```python
from build123d import *

# Parameters (mm, degrees)
SKETCH1_W               = 38.1
SKETCH1_H               = 15.875
BOSS_EXTRUDE1_DEPTH     = 7.62
SKETCH3_R               = 1.7
CUT_EXTRUDE1_DEPTH      = 49.4665
CUT_EXTRUDE2_DEPTH      = 3.302
CUT_EXTRUDE2_DEPTH_BACK = 22.2885
SKETCH4_R               = 1.7272


with BuildPart() as part:
    # Sketch1 → Boss-Extrude1 (new body)
    with BuildSketch(Plane.YZ):
        Rectangle(SKETCH1_W, SKETCH1_H)
    extrude(amount=BOSS_EXTRUDE1_DEPTH)

    # Sketch3 → Cut-Extrude1 (cut)
    with BuildSketch(Plane.XZ.offset(19.05)):
        with Locations(Location((4.36625, 0, 0), (0, 0, 270))):
            Circle(SKETCH3_R)
    extrude(amount=-CUT_EXTRUDE1_DEPTH, mode=Mode.SUBTRACT)

    # Sketch4 → Cut-Extrude2 (cut, two sides: drawn at the far end of the back side and taken through both)
    with BuildSketch(Plane.YZ.offset(7.62).offset(-CUT_EXTRUDE2_DEPTH_BACK)):
        with Locations(Location((-12.7, 4.7625, 0), (0, 0, 270))):
            Circle(SKETCH4_R)
        with Locations(Location((12.7, -4.7625, 0), (0, 0, 270))):
            Circle(SKETCH4_R)
    extrude(amount=CUT_EXTRUDE2_DEPTH + CUT_EXTRUDE2_DEPTH_BACK, mode=Mode.SUBTRACT)


solid = part.part
```
Part model, mm, in its own coordinate system. Round coordinates to 2 decimals unless told otherwise and drop trailing zeros. Write each loop counter-clockwise with the first axis right and the second up, starting at its lowest first coordinate (ties: lowest second). Pieces come first, ordered by that corner, then holes. Notation, with made-up numbers: (35.5, -9.75) -> (49.5, -9.75) arc R19 cw to (49.5, -0.75) -> close; hole circle Ø8 at (26.5, -9). An arc over 180 degrees is marked (long way). Return JSON: item names as keys, results as strings. Group by question number.
Q1. Saw through at C-C on z = 0. Write the cut outline in (x, y), plus the area to 3 significant figures.
Q2. Saw through at A-A on x = 5. Write the cut outline in (y, z), plus the area to 3 significant figures.
Q3. Mould opens along X. For faces 1 (the flat face through (7.62, 0, 0)), 2 (the flat face through (4, 0, 7.938)), 3 (the flat face through (0, 0, 0)), 4 (the cylindrical face through (5.52, -0.27, 1.25)) say: pulls with the +X half, pulls with the -X half, needs draft (parallel to the pull), parting line crosses it, or undercut.
Q4. Saw through at B-B on y = -11.5. Write the cut outline in (x, z), plus the area to 3 significant figures.
Q5. Saw through at D-D on x = 3.5. Write the cut outline in (y, z).
Q6. Probe L1, parallel to X at y = 7.5, z = 0; L2, parallel to Z at x = 5, y = 12.7; L3, parallel to Z at x = 4.5, y = -7. List the from-to ranges inside material, lowest first. Write a range as [from, to].
Answer:
{
 "1": {"outline": "(0, -19.05) -> (2.67, -19.05) -> (2.67, 19.05) -> (0, 19.05) -> close; (6.07, -19.05) -> (7.62, -19.05) -> (7.62, 19.05) -> (6.07, 19.05) -> close", "area": "161 mm2"},
 "2": {"outline": "(-19.05, -7.94) -> (19.05, -7.94) -> (19.05, -1.58) -> (-19.05, -1.58) -> close; (-19.05, 1.58) -> (19.05, 1.58) -> (19.05, 7.94) -> (-19.05, 7.94) -> close; hole circle Ø3.45 at (-12.7, 4.76); hole circle Ø3.45 at (12.7, -4.76)", "area": "466 mm2"},
 "3": {"face 1": "pulls with the +X half", "face 2": "needs draft", "face 3": "pulls with the -X half", "face 4": "undercut"},
 "4": {"outline": "(0, -7.94) -> (7.62, -7.94) -> (7.62, 3.52) -> (0, 3.52) -> close; (0, 6) -> (7.62, 6) -> (7.62, 7.94) -> (0, 7.94) -> close; hole circle Ø3.4 at (4.37, 0)", "area": "93.0 mm2"},
 "5": {"outline": "(-19.05, -7.94) -> (19.05, -7.94) -> (19.05, -1.46) -> (-19.05, -1.46) -> close; (-19.05, 1.46) -> (19.05, 1.46) -> (19.05, 7.94) -> (-19.05, 7.94) -> close; hole circle Ø3.45 at (-12.7, 4.76); hole circle Ø3.45 at (12.7, -4.76)"},
 "6": {"L1": "[0, 2.67], [6.07, 7.62]", "L2": "[-7.94, -6.49], [-3.04, -1.58], [1.58, 7.94]", "L3": "[-7.94, -1.69], [1.69, 7.94]"}
}
